The listing builds one solid part. Answer for the finished solid, in the listing's coordinates (mm). Face numbers are marked on the shaded views. A direction names the side the tool comes from. Coordinates: 2 decimals unless noted, no trailing zeros. Order: outer loops, then holes, each group sorted by start corner. A loop starts at its lowest first (then second) coordinate and runs counter-clockwise, first axis right, second up.
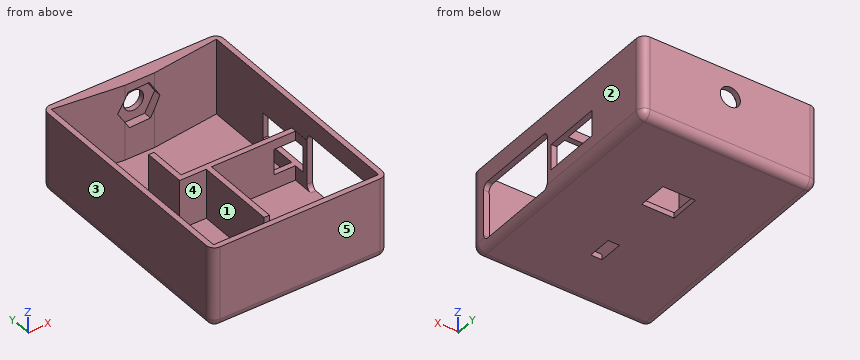
from build123d import *

# Parameters (mm, degrees)
SKETCH_1_W               = 65
SKETCH_1_H               = 30
EXTRUDE_1_DEPTH          = 88
SKETCH_4_W               = 2
SKETCH_4_H               = 40
CUT_EXTRUDE_1_DEPTH      = 28
CUT_EXTRUDE_2_DEPTH      = 6
SKETCH_7_W               = 4.182275868
SKETCH_7_H               = 9
CUT_EXTRUDE_3_DEPTH      = 6
SKETCH_8_W               = 12
SKETCH_8_H               = 11
CUT_EXTRUDE_4_DEPTH      = 6
FILLET_1_R               = 3
CUT_EXTRUDE_5_DEPTH      = 3
CUT_EXTRUDE_6_DEPTH      = 15
CUT_EXTRUDE_6_DEPTH_BACK = 6
SKETCH_12_W              = 10
SKETCH_12_H              = 9.5034376
CUT_EXTRUDE_8_DEPTH      = 5
CUT_EXTRUDE_8_DEPTH_BACK = 10
SKETCH_18_R              = 3.7
SKETCH_19_W              = 9.664954626
SKETCH_19_H              = 76.096771223
CUT_EXTRUDE_9_DEPTH      = 61


with BuildPart() as part:
    # 草图1 → 凸台-拉伸1 (new body)
    with BuildSketch(Plane(origin=(0, 0, 0), x_dir=(1, 0, 0), z_dir=(0, 1, 0))):
        Rectangle(SKETCH_1_W, SKETCH_1_H)
    extrude(amount=EXTRUDE_1_DEPTH)

    # 草图4 → 切除-拉伸1 (cut)
    with BuildSketch(Plane.XY.offset(15)):
        Polygon((-30.5, 86), (-30.5, 2), (-18.5, 2), (-9.5, 2), (30.439417497, 2), (30.439417497, 45), (-0.560582503, 45), (-0.560582503, 15), (-2.560582503, 15), (-2.560582503, 44.909852699), (-12.396150881, 44.909852699), (-12.396150881, 61), (-10.396150881, 61), (-10.396150881, 47), (24.5, 47), (30.5, 47), (30.5, 48.635726891), (30.5, 59.903593532), (30.5, 86), (5.5, 83), (-5.5, 83), align=None)
        with Locations((-25.206585503, 31)):
            Rectangle(SKETCH_4_W, SKETCH_4_H, mode=Mode.SUBTRACT)
    extrude(amount=-CUT_EXTRUDE_1_DEPTH, mode=Mode.SUBTRACT)

    # 草图6 → 切除-拉伸2 (cut)
    with BuildSketch(Plane(origin=(32.5, 0, 0), x_dir=(0, 0, -1), z_dir=(1, 0, 0))):
        with BuildLine():
            Line((13, 37), (13, 8))
            ThreePointArc((13, 8), (12.414213562, 6.585786438), (11, 6))
            Line((11, 6), (-6, 6))
            ThreePointArc((-6, 6), (-7.414213562, 6.585786438), (-8, 8))
            Line((-8, 8), (-8, 37))
            ThreePointArc((-8, 37), (-7.414213562, 38.414213562), (-6, 39))
            Line((-6, 39), (11, 39))
            ThreePointArc((11, 39), (12.414213562, 38.414213562), (13, 37))
        make_face()
    extrude(amount=-CUT_EXTRUDE_2_DEPTH, mode=Mode.SUBTRACT)

    # 草图7 → 切除-拉伸3 (cut)
    with BuildSketch(Plane.XY.offset(-13)):
        with Locations((1.530555431, 25.5)):
            Rectangle(SKETCH_7_W, SKETCH_7_H)
    extrude(amount=-CUT_EXTRUDE_3_DEPTH, mode=Mode.SUBTRACT)

    # 草图8 → 切除-拉伸4 (cut)
    with BuildSketch(Plane.XY.offset(-13)):
        with Locations((0, 56.224480757)):
            Rectangle(SKETCH_8_W, SKETCH_8_H)
    extrude(amount=-CUT_EXTRUDE_4_DEPTH, mode=Mode.SUBTRACT)

    # 圆角1
    # the kernel refuses this fillet: 3 mm, written as the material it takes off along each edge
    with BuildSketch(Plane(origin=(29.5, 3, -12), x_dir=(0, -1, 0), z_dir=(0, 0, -1))) as fillet_1_piece_1_section:
        Polygon((0, 0), (FILLET_1_R, 0), (FILLET_1_R, -FILLET_1_R), (0, -FILLET_1_R), align=None)
    fillet_1_piece_1 = extrude(amount=FILLET_1_R, mode=Mode.PRIVATE)
    fillet_1_piece_1 = fillet_1_piece_1 - Plane(origin=(29.5, 3, -12), x_dir=(-0.7071067811865475, 0.7071067811865475, 0), z_dir=(0, 0, -1)) * Sphere(FILLET_1_R, mode=Mode.PRIVATE)
    add(fillet_1_piece_1, mode=Mode.SUBTRACT)
    with BuildSketch(Plane(origin=(29.5, 85, -12), x_dir=(0, 1, 0), z_dir=(0, 0, -1))) as fillet_1_piece_2_section:
        Polygon((0, 0), (FILLET_1_R, 0), (FILLET_1_R, FILLET_1_R), (0, FILLET_1_R), align=None)
    fillet_1_piece_2 = extrude(amount=FILLET_1_R, mode=Mode.PRIVATE)
    fillet_1_piece_2 = fillet_1_piece_2 - Plane(origin=(29.5, 85, -12), x_dir=(-0.7071067811865475, -0.7071067811865475, 0), z_dir=(0, 0, -1)) * Sphere(FILLET_1_R, mode=Mode.PRIVATE)
    add(fillet_1_piece_2, mode=Mode.SUBTRACT)
    with BuildSketch(Plane(origin=(-29.5, 3, -12), x_dir=(-1, 0, 0), z_dir=(0, 0, -1))) as fillet_1_piece_3_section:
        Polygon((0, 0), (FILLET_1_R, 0), (FILLET_1_R, -FILLET_1_R), (0, -FILLET_1_R), align=None)
    fillet_1_piece_3 = extrude(amount=FILLET_1_R, mode=Mode.PRIVATE)
    fillet_1_piece_3 = fillet_1_piece_3 - Plane(origin=(-29.5, 3, -12), x_dir=(0.7071067811865475, 0.7071067811865475, 0), z_dir=(0, 0, -1)) * Sphere(FILLET_1_R, mode=Mode.PRIVATE)
    add(fillet_1_piece_3, mode=Mode.SUBTRACT)
    with BuildSketch(Plane(origin=(-29.5, 85, -12), x_dir=(-1, 0, 0), z_dir=(0, 0, -1))) as fillet_1_piece_4_section:
        Polygon((0, 0), (FILLET_1_R, 0), (FILLET_1_R, FILLET_1_R), (0, FILLET_1_R), align=None)
    fillet_1_piece_4 = extrude(amount=FILLET_1_R, mode=Mode.PRIVATE)
    fillet_1_piece_4 = fillet_1_piece_4 - Plane(origin=(-29.5, 85, -12), x_dir=(0.7071067811865475, -0.7071067811865475, 0), z_dir=(0, 0, -1)) * Sphere(FILLET_1_R, mode=Mode.PRIVATE)
    add(fillet_1_piece_4, mode=Mode.SUBTRACT)
    with BuildSketch(Plane(origin=(32.5, 3, -15), x_dir=(-1, 0, 0), z_dir=(0, 1, 0))) as fillet_1_piece_5:
        with BuildLine():
            CenterArc((FILLET_1_R, FILLET_1_R), FILLET_1_R, 180, 90)
            Line((0, FILLET_1_R), (0, 0))
            Line((0, 0), (FILLET_1_R, 0))
        make_face()
    extrude(amount=82, mode=Mode.SUBTRACT)
    with BuildSketch(Plane(origin=(-32.5, 3, -15), x_dir=(1, 0, 0), z_dir=(0, 1, 0))) as fillet_1_piece_6:
        with BuildLine():
            CenterArc((FILLET_1_R, -FILLET_1_R), FILLET_1_R, 90, 90)
            Line((0, -FILLET_1_R), (0, 0))
            Line((0, 0), (FILLET_1_R, 0))
        make_face()
    extrude(amount=82, mode=Mode.SUBTRACT)
    with BuildSketch(Plane(origin=(-32.5, 0, 22.5), x_dir=(0, 1, 0), z_dir=(0, 0, -1)), Plane(origin=(32.5, 88, -12), x_dir=(-1, 0, 0), z_dir=(0, 0, 1))) as fillet_1_piece_7:
        with BuildLine():
            CenterArc((FILLET_1_R, FILLET_1_R), FILLET_1_R, 180, 90)
            Line((0, FILLET_1_R), (0, 0))
            Line((0, 0), (FILLET_1_R, 0))
        make_face()
    extrude(amount=34.5, mode=Mode.SUBTRACT)
    with BuildSketch(Plane(origin=(32.5, 0, -12), x_dir=(-1, 0, 0), z_dir=(0, 0, 1)), Plane(origin=(-32.5, 88, 22.5), x_dir=(0, -1, 0), z_dir=(0, 0, -1))) as fillet_1_piece_8:
        with BuildLine():
            CenterArc((FILLET_1_R, -FILLET_1_R), FILLET_1_R, 90, 90)
            Line((0, -FILLET_1_R), (0, 0))
            Line((0, 0), (FILLET_1_R, 0))
        make_face()
    extrude(amount=34.5, mode=Mode.SUBTRACT)
    with BuildSketch(Plane(origin=(-29.5, 0, -15), x_dir=(0, 1, 0), z_dir=(1, 0, 0))) as fillet_1_piece_9:
        with BuildLine():
            CenterArc((FILLET_1_R, FILLET_1_R), FILLET_1_R, 180, 90)
            Line((0, FILLET_1_R), (0, 0))
            Line((0, 0), (FILLET_1_R, 0))
        make_face()
    extrude(amount=59, mode=Mode.SUBTRACT)
    with BuildSketch(Plane(origin=(-29.5, 88, -15), x_dir=(0, -1, 0), z_dir=(1, 0, 0))) as fillet_1_piece_10:
        with BuildLine():
            CenterArc((FILLET_1_R, -FILLET_1_R), FILLET_1_R, 90, 90)
            Line((0, -FILLET_1_R), (0, 0))
            Line((0, 0), (FILLET_1_R, 0))
        make_face()
    extrude(amount=59, mode=Mode.SUBTRACT)

    # 草图10 → 切除-拉伸5 (cut)
    with BuildSketch(Plane.XZ.offset(-83)):
        Polygon((3.993436667, -1.290973026), (7.651958762, 5.591266151), (3.521025848, 12.200758813), (-4.268429161, 11.9280123), (-7.926951256, 5.045773123), (-3.796018342, -1.563719539), align=None)
    extrude(amount=-CUT_EXTRUDE_5_DEPTH, mode=Mode.SUBTRACT)

    # 草图12 → 切除-拉伸6 (cut, two sides: drawn at the far end of the back side and taken through both)
    with BuildSketch(Plane(origin=(0, 47, 0), x_dir=(1, 0, 0), z_dir=(0, 1, 0)).offset(-CUT_EXTRUDE_6_DEPTH_BACK)):
        with Locations((27.504184345, 2.8493686)):
            Rectangle(SKETCH_12_W, SKETCH_12_H)
    extrude(amount=CUT_EXTRUDE_6_DEPTH + CUT_EXTRUDE_6_DEPTH_BACK, mode=Mode.SUBTRACT)

    # 草图18 → 切除-拉伸8 (cut, two sides: drawn at the far end of the back side and taken through both)
    with BuildSketch(Plane.XZ.offset(-83).offset(-CUT_EXTRUDE_8_DEPTH_BACK)):
        with Locations(Location((-0.137496247, 5.318519637, 0), (0, 0, 90))):
            Circle(SKETCH_18_R)
    extrude(amount=CUT_EXTRUDE_8_DEPTH + CUT_EXTRUDE_8_DEPTH_BACK, mode=Mode.SUBTRACT)

    # 草图19 → 切除-拉伸9 (cut)
    with BuildSketch(Plane(origin=(-30.5, 0, 0), x_dir=(0, 0, -1), z_dir=(1, 0, 0))):
        with Locations((-10.167522687, 40.608730848)):
            Rectangle(SKETCH_19_W, SKETCH_19_H)
    extrude(amount=CUT_EXTRUDE_9_DEPTH, mode=Mode.SUBTRACT)


solid = part.part
1) A tool of negligible diameter and unlimited length cuts with its end or side. For the marked faces 1 and 2, from which of +Z, -Z, +X, -X, +Y, -Y can it reach the whole face along a straight path? Write none if from no direction.
2) Section D-D (y = 54) is taken. Give the vertices of the cut face in (x, z).
3) Each of these flat-tipped pins is pushed along its axis until it touches: P1, Ø1, axis at x = -6.5, z = -10.5, coming from the -Y side; P2, Ø0.6, axis at x = -1, z = -14.5, coming from the -Y side; P3, Ø1, axis at x = -25, y = 33.5, coming from the +Z side; P4, Ø4, axis at y = 56, z = -0.5, coming from the +X side. Where does it stop, or does it pass through?
4) Consider L1, parallel to X at y = 22, z = -10; L2, parallel to X at y = 60, z = 12.5; L3, parallel to X at y = 4.5, z = 0.5. Determine where each line is inside the solid, lowest interval first.
5) Section A-A (y = 31) is taken. Give the vertices of the cut face in (x, z), then the cut area to 3 significant figures.
6) Section B-B (x = 24) is taken. Give the vertices of the cut face in (y, z), then the cut area to 3 significant figures.
7) Determine the mould class of the marked faces 3, 4 and 5 for opening direction X: released by +X, released by -X, zero draft, split by the parting line, or undercut.
Filled sheet:
1. face 1: +Z
1. face 2: +Z, -Z, +X, +Y, -Y
2. outline: (-32.5, -12) arc R3 ccw to (-29.5, -15) - (-6, -15) - (-6, -13) - (-10.4, -13) - (-10.4, 5.34) - (-12.4, 5.34) - (-12.4, -13) - (-30.5, -13) - (-30.5, 15) - (-32.5, 15) - close; (6, -15) - (29.5, -15) arc R3 ccw to (32.5, -12) - (32.5, -7.6) - (30.5, -7.6) - (30.5, -13) - (6, -13) - close; (30.5, 1.9) - (32.5, 1.9) - (32.5, 15) - (30.5, 15) - close
3. P1: stops at y = 0
3. P2: stops at y = 0.96
3. P3: stops at z = 5.34
3. P4: stops at x = -10.4
4. L1: x = -32.5 to -30.5, -26.21 to -24.21, -2.56 to -0.56
4. L2: x = -32.5 to -30.5, 30.5 to 32.5
4. L3: x = -32.5 to -30.5, 30.44 to 32.5
5. outline: (-32.5, -12) arc R3 ccw to (-29.5, -15) - (29.5, -15) arc R3 ccw to (32.33, -13) - (-0.56, -13) - (-0.56, 5.34) - (-2.56, 5.34) - (-2.56, -13) - (-24.21, -13) - (-24.21, 5.34) - (-26.21, 5.34) - (-26.21, -13) - (-30.5, -13) - (-30.5, 15) - (-32.5, 15) - close; (30.5, 8) - (32.5, 8) - (32.5, 15) - (30.5, 15) - close
5. area: 270 mm2
6. outline: (0, -12) arc R3 ccw to (3, -15) - (85, -15) arc R3 ccw to (88, -12) - (88, 15) - (85.22, 15) - (85.22, -13) - (47, -13) - (47, -7.6) - (45, -7.6) - (45, -13) - (2, -13) - (2, 15) - (0, 15) - close; (45, 1.9) - (47, 1.9) - (47, 5.34) - (45, 5.34) - close
6. area: 324 mm2
7. face 3: released by -X
7. face 4: undercut
7. face 5: zero draft
